```python
from build123d import *

# Parameters (mm, degrees)
SKETCH1_W           = 140
SKETCH1_H           = 120
SKETCH1_W_2         = 131
SKETCH1_H_2         = 111
BOSS_EXTRUDE1_DEPTH = 16
CUT_EXTRUDE1_DEPTH  = 186.08376482
SKETCH5_R           = 1.25
CUT_EXTRUDE3_DEPTH  = 186.08376482
CUT_EXTRUDE2_DEPTH  = 186.08376482
BOSS_EXTRUDE2_DEPTH = 115.5
SKETCH7_W           = 136
SKETCH7_H           = 108
CUT_EXTRUDE4_DEPTH  = 186.08376482
FILLET1_R           = 2
SKETCH9_R           = 1.3
CUT_EXTRUDE5_DEPTH  = 4
SKETCH10_R          = 1.5
CUT_EXTRUDE6_DEPTH  = 186.08376482


with BuildPart() as part:
    # Sketch1 → Boss-Extrude1 (new body)
    with BuildSketch(Plane(origin=(0, 0, 0), x_dir=(1, 0, 0), z_dir=(0, 1, 0))):
        with Locations((-70, 60)):
            Rectangle(SKETCH1_W, SKETCH1_H)
        with Locations((-70, 60)):
            Rectangle(SKETCH1_W_2, SKETCH1_H_2, mode=Mode.SUBTRACT)
    extrude(amount=BOSS_EXTRUDE1_DEPTH)

    # Sketch3 → Cut-Extrude1 (cut, through all)
    with BuildSketch(Plane.XY):
        with BuildLine():
            Line((-129.15, 8), (-129.15, 0))
            Line((-129.15, 0), (-125.15, 0))
            Line((-125.15, 0), (-125.15, 8))
            ThreePointArc((-125.15, 8), (-127.15, 10), (-129.15, 8))
        make_face()
        with BuildLine():
            Line((-14.85, 8), (-14.85, 0))
            Line((-14.85, 0), (-10.85, 0))
            Line((-10.85, 0), (-10.85, 8))
            ThreePointArc((-10.85, 8), (-12.85, 10), (-14.85, 8))
        make_face()
    extrude(amount=-CUT_EXTRUDE1_DEPTH, mode=Mode.SUBTRACT)

    # Sketch5 → Cut-Extrude3 (cut, through all)
    with BuildSketch(Plane.XY):
        with Locations((-132.65, 8)):
            Circle(SKETCH5_R)
        with Locations((-121.65, 8)):
            Circle(SKETCH5_R)
        with Locations((-18.35, 8)):
            Circle(SKETCH5_R)
        with Locations((-7.35, 8)):
            Circle(SKETCH5_R)
    extrude(amount=-CUT_EXTRUDE3_DEPTH, mode=Mode.SUBTRACT)

    # Sketch4 → Cut-Extrude2 (cut, through all)
    with BuildSketch(Plane(origin=(0, 16, 0), x_dir=(1, 0, 0), z_dir=(0, 1, 0))):
        Polygon((-138, 115.5), (-118.5, 115.5), (-118.5, 118), (-21.5, 118), (-21.5, 115.5), (-2, 115.5), (-2, 4.5), (-21.5, 4.5), (-21.5, 2), (-118.5, 2), (-118.5, 4.5), (-138, 4.5), align=None)
    extrude(amount=-CUT_EXTRUDE2_DEPTH, mode=Mode.SUBTRACT)

    # Sketch6 → Boss-Extrude2 (add)
    with BuildSketch(Plane.XY):
        with BuildLine():
            Line((-140, 16), (-135, 16))
            Line((-135, 16), (-135, 11.259984663))
            ThreePointArc((-135, 11.259984663), (-135.65, 8), (-135, 4.740015337))
            Line((-135, 4.740015337), (-135, 0))
            Line((-135, 0), (-140, 0))
            Line((-140, 0), (-140, 16))
        make_face()
        with BuildLine():
            Line((-5, 16), (-5, 11.259984663))
            ThreePointArc((-5, 11.259984663), (-4.35, 8), (-5, 4.740015337))
            Line((-5, 4.740015337), (-5, 0))
            Line((-5, 0), (0, 0))
            Line((0, 0), (0, 16))
            Line((0, 16), (-5, 16))
        make_face()
    extrude(amount=-BOSS_EXTRUDE2_DEPTH)

    # Sketch7 → Cut-Extrude4 (cut, through all)
    with BuildSketch(Plane(origin=(0, 16, 0), x_dir=(1, 0, 0), z_dir=(0, 1, 0))):
        with Locations((-70, 60)):
            Rectangle(SKETCH7_W, SKETCH7_H)
    extrude(amount=-CUT_EXTRUDE4_DEPTH, mode=Mode.SUBTRACT)

    # Fillet1
    fillet1_edges = [part.edges().sort_by_distance(p)[0] for p in [
        (-118.5, 8, -118),
        (-21.5, 8, -118),
        (-21.5, 8, -2),
        (-118.5, 8, -2),
        (-2, 8, -6),
        (-138, 8, -6),
        (-138, 8, -114),
        (-2, 8, -114),
    ]]
    fillet(fillet1_edges, radius=FILLET1_R)

    # Sketch9 → Cut-Extrude5 (cut)
    with BuildSketch(Plane(origin=(0, 0, 0), x_dir=(1, 0, 0), z_dir=(0, 1, 0))):
        with Locations(Location((-137.25, 2.75, 0), (0, 0, 270))):
            Circle(SKETCH9_R)
        with Locations(Location((-2.75, 2.75, 0), (0, 0, 90))):
            Circle(SKETCH9_R)
        with Locations(Location((-2.75, 117.25, 0), (0, 0, 270))):
            Circle(SKETCH9_R)
        with Locations(Location((-137.25, 117.25, 0), (0, 0, 90))):
            Circle(SKETCH9_R)
    extrude(amount=CUT_EXTRUDE5_DEPTH, mode=Mode.SUBTRACT)

    # Sketch10 → Cut-Extrude6 (cut, through all)
    with BuildSketch(Plane(origin=(0, 16, 0), x_dir=(1, 0, 0), z_dir=(0, 1, 0))):
        with Locations(Location((-137.25, 117.25, 0), (0, 0, 270))):
            Circle(SKETCH10_R)
        with Locations(Location((-2.75, 117.25, 0), (0, 0, 90))):
            Circle(SKETCH10_R)
        with Locations(Location((-2.75, 2.75, 0), (0, 0, 270))):
            Circle(SKETCH10_R)
        with Locations(Location((-137.25, 2.75, 0), (0, 0, 90))):
            Circle(SKETCH10_R)
    extrude(amount=-CUT_EXTRUDE6_DEPTH, mode=Mode.SUBTRACT)


solid = part.part
```
The model under review builds one solid part; all positions refer to its coordinate system, in mm. A direction names the side the tool comes from. Coordinates: 2 decimals unless noted, no trailing zeros. Write each loop counter-clockwise with the first axis right and the second up, starting at its lowest first coordinate (ties: lowest second). Pieces come first, ordered by that corner, then holes. Notation, with made-up numbers: (77, -23) - (97, -23) arc R17 ccw to (97, -11) - close; hole circle Ø1 at (43, 26.25). An arc over 180 degrees is marked (long way). Answer in a Markdown table with one row per item. Add a question column.
Q1. Consider section A-A on z = -62. Give the boundary of the cut face in (x, y).
Q2. For faces 4 (the face through (-125.15, 4, -118)), 5 (the face through (-71, 0, -119)), 6 (the face through (-71, 8, -118)), list the 3-axis set-ups (+Z, -Z, +X, -X, +Y, -Y) from which the entire face can be reached by the end or side of a thin tool; tool diameter is ignored.
Q3. Consider section C-C on y = 2. Give the number of separate pieces and of enclosed holes in the cut face, then the cut area to 3 significant figures.
Q4. To check wall thickness, follow line 1 along X through (y, z) = (3.75, -82); line 2 along Z through (x, y) = (-51.5, 9.75); line 3 along Z through (x, y) = (-131.5, 12.5). State the ranges of each line that lie inside material, in increasing order. Write a range as from..to.
Q5. Clearance check with flat-ended pins moving along their axes: pin 1 (1.5 mm diameter, centred on x = -7.35, y = 8, fed in from -Z); pin 2 (4 mm diameter, centred on x = -2.75, z = -2.75, fed in from +Y). State where each tip first meets the part, or that it passes through.
Q6. Draft analysis for pull direction Z (two halves, no side actions). For faces 1 (the face through (-136.24, 8.11, -118.36)), 2 (the face through (-10.85, 4, -118)), 3 (the face through (-71, 8, 0)), state which applies: +Z half, -Z half, draft (parallel to the pull), parting line (faces both ways), or undercut.
Q7. Consider section B-B on x = -50. Give the boundary of the cut face in (y, z).
Answers below:
| question | item | result |
|---|---|---|
| 1 | outline | (-140, 0) - (-138, 0) - (-138, 16) - (-140, 16) - close; (-2, 0) - (0, 0) - (0, 16) - (-2, 16) - close |
| 2 | face 4 | +Z, -Z, -Y |
| 2 | face 5 | +Z, -Z, +X, -X, -Y |
| 2 | face 6 | +Y, -Y |
| 3 | separate pieces | 4 |
| 3 | enclosed holes | 4 |
| 3 | area | 1,140 mm² |
| 4 | line 1 | -140..-138, -2..0 |
| 4 | line 2 | -120..-118, -2..0 |
| 4 | line 3 | -120..-115.5, -4.5..0 |
| 5 | pin 1 | through |
| 5 | pin 2 | y = 16 |
| 6 | face 1 | undercut |
| 6 | face 2 | draft |
| 6 | face 3 | +Z half |
| 7 | outline | (0, -120) - (16, -120) - (16, -118) - (0, -118) - close; (0, -2) - (16, -2) - (16, 0) - (0, 0) - close |
